Build history of the part. All positions in model axes, mm. Face numbers are marked on the shaded views. A direction names the side the tool comes from. Give positions to 0.01 mm unless a question says otherwise; leave off trailing zeros. Use a Markdown table: item, result.
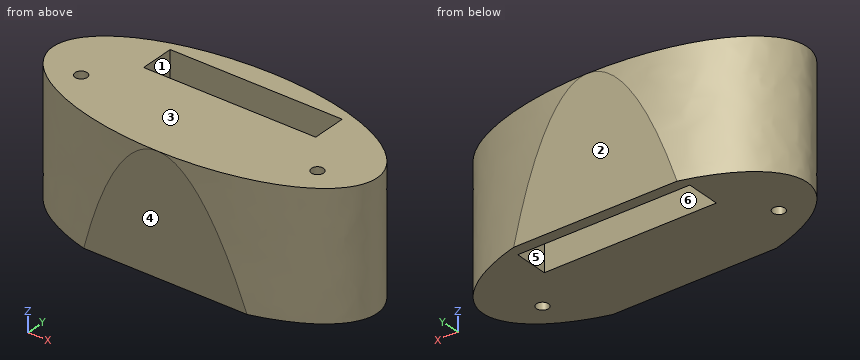
from build123d import *

# Parameters (mm, degrees)
SKETCH1_RX              = 240
SKETCH1_RY              = 110
BOSS_EXTRUDE1_DEPTH     = 186.33
SKETCH10_W              = 254.8
SKETCH10_H              = 50.8
CUT_EXTRUDE5_DEPTH      = 324.139085999
SKETCH12_R              = 9
CUT_EXTRUDE8_DEPTH      = 324.139085999
CUT_EXTRUDE9_DEPTH      = 324.139085999
CUT_EXTRUDE9_DEPTH_BACK = 324.139085999


with BuildPart() as part:
    # Sketch1 → Boss-Extrude1 (new body)
    with BuildSketch(Plane.XY):
        with Locations((0, 0)):
            Ellipse(SKETCH1_RX, SKETCH1_RY)
    extrude(amount=-BOSS_EXTRUDE1_DEPTH)

    # Sketch10 → Cut-Extrude5 (cut, through all)
    with BuildSketch(Plane.XY):
        with Locations((0, 53.5)):
            Rectangle(SKETCH10_W, SKETCH10_H)
    extrude(amount=-CUT_EXTRUDE5_DEPTH, mode=Mode.SUBTRACT)

    # Sketch12 → Cut-Extrude8 (cut, through all)
    with BuildSketch(Plane.XY):
        with Locations((175, -30)):
            Circle(SKETCH12_R)
        with Locations(Location((-175, -30, 0), (0, 0, 180))):
            Circle(SKETCH12_R)
    extrude(amount=-CUT_EXTRUDE8_DEPTH, mode=Mode.SUBTRACT)

    # Sketch14 → Cut-Extrude9 (cut, two sides: drawn at the far end of the back side and taken through both)
    with BuildSketch(Plane(origin=(0, 0, 0), x_dir=(0, 0, -1), z_dir=(1, 0, 0)).offset(-CUT_EXTRUDE9_DEPTH_BACK)):
        Polygon((0, 110), (186.33, 95), (186.33, 110), align=None)
        Polygon((0, -110), (186.33, -95), (186.33, -110), align=None)
    extrude(amount=CUT_EXTRUDE9_DEPTH + CUT_EXTRUDE9_DEPTH_BACK, mode=Mode.SUBTRACT)


solid = part.part
1) Two-plate mould, pull along Y, no slides. Class the marked faces 3, 4, 5 and 6: +Y half, -Y half, draft (parallel to the pull), parting line (faces both ways), or undercut.
Computed:
| item | result |
|---|---|
| face 3 | draft |
| face 4 | -Y half |
| face 5 | undercut |
| face 6 | undercut |
2) Wall check: line 1 (X direction, y = 55.5, z = -68.5); line 2 (Y direction, x = -175, z = -38); line 3 (X direction, y = 29, z = -13). Give the ranges that are in metal, low to high. Write a range as from..to.
Computed:
| item | result |
|---|---|
| line 1 | x = -207.21..-127.4, 127.4..207.21 |
| line 2 | y = -75.28..-39, -21..75.28 |
| line 3 | x = -231.51..-127.4, 127.4..231.51 |
3) Pin check, flat tips, straight feed: P1, Ø1.5, axis at y = 25, z = -81, coming from the -X side; P2, Ø1.5, axis at x = 140.5, z = -158.5, coming from the -Y side; P3, Ø14.5, axis at x = -175, y = -30, coming from the +Z side; P4, Ø12, axis at x = -36.5, z = -101.5, coming from the -Y side. Stop position of each tip, or through.
Computed:
| item | result |
|---|---|
| P1 | stops at x = -234.1 |
| P2 | stops at y = -89.43 |
| P3 | passes through |
| P4 | stops at y = -102.31 |
4) Tool access for the marked faces 1 and 2: list every direction of +Z, -Z, +X, -X, +Y, -Y with a clear straight run to the whole face (end or side of a thin tool).
Computed:
| item | result |
|---|---|
| face 1 | +Z, -Z |
| face 2 | -Z, +X, -X, +Y |
5) Slice it at A-A (y = -30). State how many separate pieces and enclosed holes the cut face has, and give its area (3 significant figures).
Computed:
| item | result |
|---|---|
| separate pieces | 3 |
| enclosed holes | 0 |
| area | 79,300 mm² |
